Could you check a few things on this drawing? It's one solid part, dimensions in mm from its lowest x, y, z. Give positions to 0.01 mm unless a question says otherwise; leave off trailing zeros. Loops run counter-clockwise (first coordinate to the right, second up) from the corner with the lowest first, then second, coordinate; pieces in that order, holes last. Notation, with made-up numbers: (31, -38.75) - (47, -38.75) arc R14 ccw to (47, -30.75) - close; hole circle Ø9 at (45, -37). An arc over 180 degrees is marked (long way). Use CSV: the item, a comma, the result in double quotes.
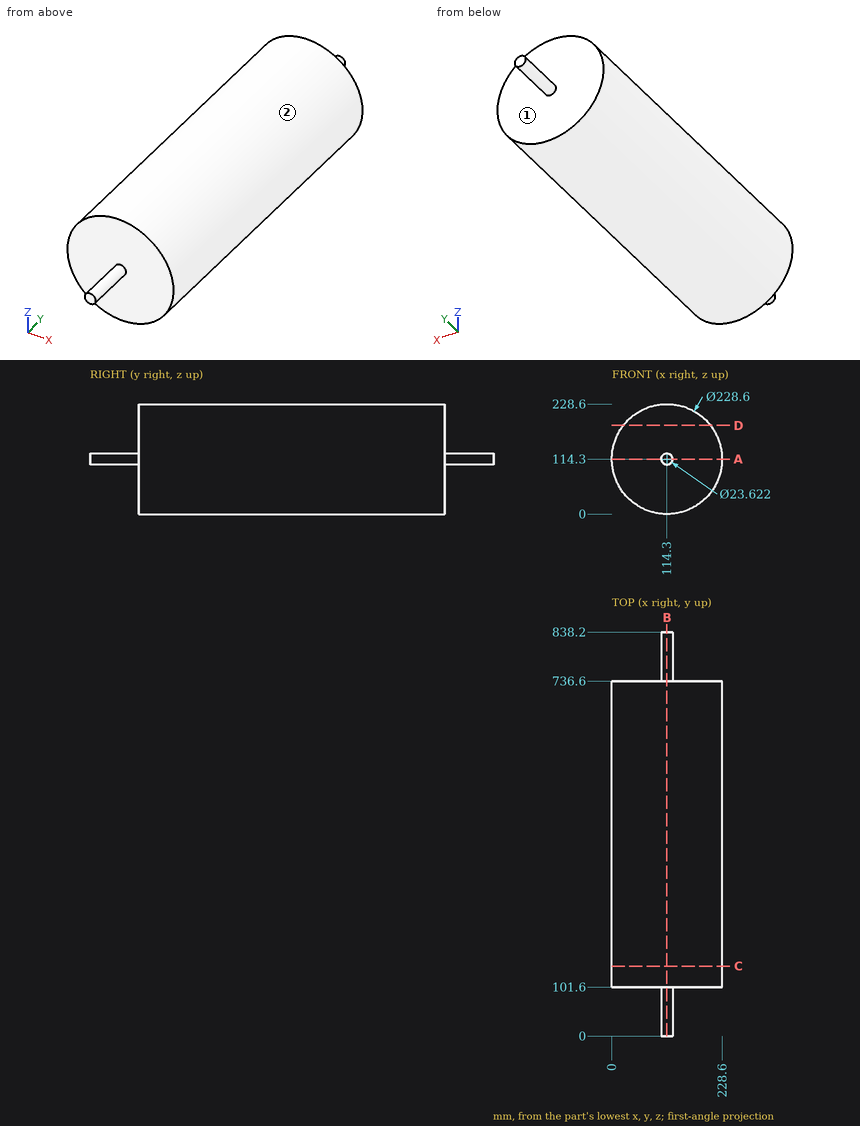
1) Suppose I cut it at B-B (x = 114.3). Please give me the cut outline in (y, z), plus the area to 3 significant figures.
Answer below:
outline,"(0, 102.49) - (101.6, 102.49) - (101.6, 0) - (736.6, 0) - (736.6, 102.49) - (838.2, 102.49) - (838.2, 126.11) - (736.6, 126.11) - (736.6, 228.6) - (101.6, 228.6) - (101.6, 126.11) - (0, 126.11) - close"
area,"150,000 mm2"
2) I need wall thicknesses on line 1 along Y through (x, z) = (69, 119.5); line 2 along X through (y, z) = (577, 127.5); line 3 along X through (y, z) = (599, 70). Which ranges of each line are inside material? Lowest first, please.
Answer below:
line 1,"y = 101.6 to 736.6"
line 2,"x = 0.76 to 227.84"
line 3,"x = 8.93 to 219.67"
3) We'd pull the mould along X, two halves only. Please class the marked faces 1 and 2: +X half, -X half, draft (parallel to the pull), parting line (faces both ways), or undercut.
Answer below:
face 1,"draft"
face 2,"parting line"
4) Suppose I cut it at D-D (z = 184). Please give me the cut outline in (x, y).
Answer below:
outline,"(23.71, 101.6) - (204.89, 101.6) - (204.89, 736.6) - (23.71, 736.6) - close"
5) Suppose I cut it at C-C (y = 145). Please give me the cut outline in (x, z).
Answer below:
outline,"circle Ø228.6 at (114.3, 114.3)"
6) Suppose I cut it at A-A (z = 114.3). Please give me the cut outline in (x, y), plus the area to 3 significant figures.
Answer below:
outline,"(0, 101.6) - (102.49, 101.6) - (102.49, 0) - (126.11, 0) - (126.11, 101.6) - (228.6, 101.6) - (228.6, 736.6) - (126.11, 736.6) - (126.11, 838.2) - (102.49, 838.2) - (102.49, 736.6) - (0, 736.6) - close"
area,"150,000 mm2"
7) I'm going to push flat-ended pins straight in: P1, Ø1, axis at x = 87.5, z = 35, coming from the +Y side; P2, Ø4, axis at y = 162.5, z = 31, coming from the +X side; P3, Ø12, axis at x = 51.5, y = 623, coming from the +Z side. Where does each tip first touch, or does it pass through?
Answer below:
P1,"stops at y = 736.6"
P2,"stops at x = 194.64"
P3,"stops at z = 213.49"
